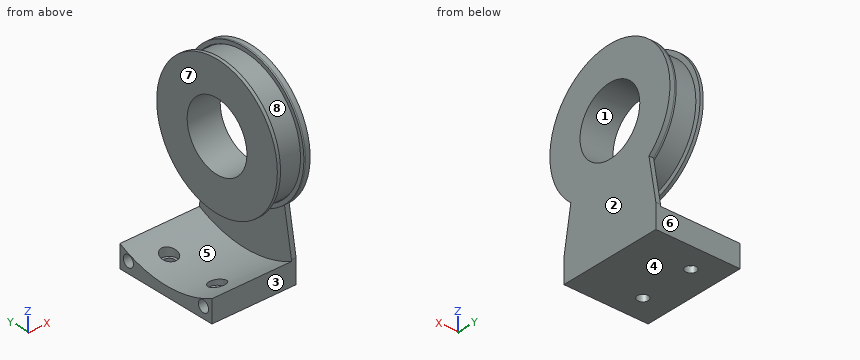
Solid Edge part; units mm, degrees
sketch "Sketch1" plane through (0, 0, 0) normal (0, 0, 1) x (1, 0, 0)
  line L0 (0, -16.3207) -> (0, 16.3207)
  line L1 (0, 16.3207) -> (26.3559, 16.3207)
  line L2 (26.3559, 16.3207) -> (26.3559, -16.3207)
  line L3 (26.3559, -16.3207) -> (0, -16.3207)
extrude "Protrusion1" add sketch "Sketch1" along normal up to vertex (7.5 mm away)
sketch "Sketch2" plane through (0, 12.45, 7.5) normal (0, 0, 1) x (1, 0, 0)
  circle A0 centre (8.5231, -3.9294) radius 2.5
  circle A1 centre (8.5233, -20.9753) radius 2.5
extrude "Cutout1" cut sketch "Sketch2" against normal blind 5.5
sketch "Sketch3" plane through (0, 0, 3.5) normal (-1, 0, 0) x (0, 0, 1)
  line L0 (4, 16.3207) -> (4, -16.3207)
  line L1 (4, -16.3207) -> (3.5, -16.3207)
  arc A0 (3.5, -16.3207) -> (3.5, 16.3207) centre (34.9133, 0) cw
  line L2 (4, 16.3207) -> (3.5, 16.3207)
extrude "Cutout2" cut sketch "Sketch3" against normal blind 24.9
sketch "Sketch4" plane through (26.3559, 27.5207, 3.5) normal (1, 0, 0) x (0, 1, 0)
  line L0 (-43.8414, 4) -> (-43.8414, -3.5)
  line L1 (-43.8414, -3.5) -> (-11.2, -3.5)
  line L2 (-11.2, -3.5) -> (-11.2, 4)
  line L3 (-11.2, 4) -> (-13.6685, 18)
  arc A0 (-41.3728, 18) -> (-13.6685, 18) centre (-27.5207, 34.1805) cw
  line L4 (-43.8414, 4) -> (-41.3728, 18)
extrude "Protrusion2" add sketch "Sketch4" against normal up to vertex (1.4559 mm away)
sketch "Sketch5" plane through (0, 13.7603, 0) normal (0, 0, -1) x (1, 0, 0)
  circle A0 centre (8.5233, 22.2857) radius 1.7
  circle A1 centre (8.5231, 5.2398) radius 1.7
extrude "Cutout3" cut sketch "Sketch5" against normal up to next
sketch "Sketch6" plane through (0, 0, 3.5) normal (-1, 0, 0) x (0, 0, 1)
  circle A0 centre (0, -13.3207) radius 1.8
  circle A1 centre (0, 13.3207) radius 1.8
extrude "Cutout4" cut sketch "Sketch6" against normal blind 7.6
sketch "Sketch7" plane through (24.9, 24.9, 30.7298) normal (-1, 0, 0) x (0, 0.1736482, 0.9848078)
  circle A0 centre (2.5213, -25.7287) radius 21.3
  circle A1 centre (2.5213, -25.7287) radius 20.1
extrude "Protrusion3" add sketch "Sketch7" along normal blind 0.5
sketch "Sketch8" plane through (24.9, 24.9, 38.9028) normal (-1, 0, 0) x (0, -1, 0)
  circle A0 centre (24.9, -1.2224) radius 19.9
extrude "Protrusion4" add sketch "Sketch8" along normal blind 7.9
sketch "Sketch9" plane through (17, 17, 38.9028) normal (-1, 0, 0) x (0, -1, 0)
  circle A0 centre (17, -1.2224) radius 21.4
extrude "Protrusion5" add sketch "Sketch9" along normal blind 1
sketch "Sketch10" plane through (26.3559, 27.5207, 10.5562) normal (1, 0, 0) x (0, 1, 0)
  circle A0 centre (-27.5207, 27.1243) radius 10.6033
extrude "Cutout5" cut sketch "Sketch10" against normal up to next
For this review, take the finished solid that the model builds, in its own axes (mm). Face numbers are marked on the shaded views. A direction names the side the tool comes from. Coordinates: 2 decimals unless noted, no trailing zeros. Loops run counter-clockwise (first coordinate to the right, second up) from the corner with the lowest first, then second, coordinate; pieces in that order, holes last.
1. Add section A-A, the plane y = 0. Give the boundary of the cut face in (x, z), then the cut area to 3 significant figures.
2. Insertion check: P1, Ø21.5, axis at y = -2.5, z = 35.5, coming from the -X side; P2, Ø2, axis at x = 15.5, z = 32.5, coming from the -Y side; P3, Ø3, axis at x = 8.52, y = -8.53, coming from the +Z side; P4, Ø4, axis at x = 23.5, z = 25.5, coming from the +Y side. Each pin has a flat end and moves straight along its axis. Give the tip position at first contact, or say it passes through.
3. Add section B-B, the plane x = 9. Give the boundary of the cut face in (y, z), then the cut area to 3 significant figures.
4. For line 1 (Z direction, x = 23.5, y = -4); line 2 (Z direction, x = 23.25, y = -6.5); line 3 (Y direction, x = 24.75, z = 56), list the stretches that pass through material, from the lowest coordinate up.
5. Add section C-C, the plane y = -9.5. Count the separate pieces of the cut face and the enclosed holes in it, then the cut area to 3 significant figures.
6. For the marked faces 4, 5, 6, 7 and 8, list the 3-axis set-ups (+Z, -Z, +X, -X, +Y, -Y) from which the entire face can be reached by the end or side of a thin tool; tool diameter is ignored.
7. Mouldability with a two-part tool opening along Y and no side actions: class the marked faces 1, 2 and 3 as +Y half, -Y half, draft (parallel to the pull), parting line (faces both ways), or undercut.
8. Add section D-D, the plane z = 55. Give the boundary of the cut face in (x, y).
Result:
1. outline: (0, 0) - (26.36, 0) - (26.36, 27.08) - (16, 27.08) - (16, 16.28) - (17, 16.28) - (17, 17.78) - (24.9, 17.78) - (24.9, 17.58) - (24.4, 17.58) - (24.4, 16.38) - (24.9, 16.38) - (24.9, 3.01) - (0, 3.01) - close; (16, 48.28) - (26.36, 48.28) - (26.36, 58.98) - (24.4, 58.98) - (24.4, 57.78) - (24.9, 57.78) - (24.9, 57.58) - (17, 57.58) - (17, 59.08) - (16, 59.08) - close
1. area: 300 mm2
2. P1: stops at x = 16
2. P2: stops at y = -20.96
2. P3: passes through
2. P4: stops at y = 18.59
3. outline: (-16.32, 0) - (-10.16, 0) - (-10.16, 2) - (-10.98, 2) - (-10.98, 4.76) arc R35.4 cw to (-16.32, 7) - close; (-6.89, 0) - (6.89, 0) - (6.89, 2) - (6.07, 2) - (6.07, 3.54) arc R35.4 cw to (-6.07, 3.54) - (-6.07, 2) - (-6.89, 2) - close; (10.15, 0) - (16.32, 0) - (16.32, 7) arc R35.4 cw to (10.97, 4.76) - (10.97, 2) - (10.15, 2) - close
3. area: 107 mm2
4. line 1: z = 0 to 3.24, 18.19 to 27.86, 47.5 to 57.17
4. line 2: z = 0 to 3.62, 18.87 to 29.3, 46.06 to 56.49
4. line 3: y = -10.87 to -8.27, -7.77 to 7.77, 8.27 to 10.87
5. separate pieces: 3
5. enclosed holes: 0
5. area: 392 mm2
6. face 4: -Z, +X, -X, +Y, -Y
6. face 5: -X
6. face 6: -Z, +X, -X, +Y
6. face 7: +Z, -X, +Y, -Y
6. face 8: none
7. face 1: undercut
7. face 2: draft
7. face 3: -Y half
8. outline: (16, -12.57) - (17, -12.57) - (17, -9.8) - (24.9, -9.8) - (24.9, -10.2) - (24.4, -10.2) - (24.4, -12.4) - (26.36, -12.4) - (26.36, 12.4) - (24.4, 12.4) - (24.4, 10.2) - (24.9, 10.2) - (24.9, 9.8) - (17, 9.8) - (17, 12.57) - (16, 12.57) - close
